For this review, take the finished solid that the model builds, in its own axes (mm). A direction names the side the tool comes from. Coordinates: 2 decimals unless noted, no trailing zeros. Write each loop counter-clockwise with the first axis right and the second up, starting at its lowest first coordinate (ties: lowest second). Pieces come first, ordered by that corner, then holes.
1) To check wall thickness, follow line 1 along Z through (x, y) = (7, 14); line 2 along Z through (x, y) = (-6, -3.5); line 3 along X through (y, z) = (-0.5, 7). State the ranges of each line that lie inside material, in increasing order.
2) Mouldability with a two-part tool opening along Z and no side actions: class faces 3 (the face through (0, 25, -71)), 4 (the face through (0, 0, 24.9)), 5 (the face through (0, 0, -143)) as pulls with the +Z half, pulls with the -Z half, needs draft (parallel to the pull), parting line crosses it, or undercut.
3) We need section B-B on y = 7. Write out the cut boundary in (x, z).
4) For faces 1 (the face through (-11, 6, 0)), 2 (the face through (-25, 0, -71)), list the 3-axis set-ups (+Z, -Z, +X, -X, +Y, -Y) from which the entire face can be reached by the end or side of a thin tool; tool diameter is ignored.
5) We need section C-C on x = 15. Write out the cut boundary in (y, z), then the cut area to 3 significant figures.
6) Insertion check: P1, Ø1, axis at y = 7, z = 2, coming from the +X side; P2, Ø1.5, axis at x = 8, y = -16.5, coming from the +Z side; P3, Ø8, axis at x = -10, z = 3.5, coming from the -Y side. Each pin has a flat end and moves straight along its axis. Give the tip position at first contact, or say it passes through.
7) We need section A-A on x = 0. Write out the cut boundary in (y, z).
Autodesk Inventor part; units mm, degrees
ref_plane "YZ Plane" through (0, 0, 0) normal (1, 0, 0) x (0, 1, 0)
ref_plane "XZ Plane" through (0, 0, 0) normal (0, 1, 0) x (-1, 0, 0)
ref_plane "XY Plane" through (0, 0, 0) normal (0, 0, 1) x (1, 0, 0)
sketch "Sketch1" plane through (0, 0, 0) normal (0, 0, 1) x (1, 0, 0)
  line L0 (-25, 25) -> (25, 25)
  line L1 (25, 25) -> (25, -25)
  line L2 (25, -25) -> (-25, -25)
  line L3 (-25, -25) -> (-25, 25)
  point P0 (0, 0)
  dimension "d0" = 50
  dimension "d1" = 50
  dimension "d2" = 25
  dimension "d3" = 25
extrude "Extrusion1" add sketch "Sketch1" against normal blind 143
sketch "Sketch2" plane through (0, 0, 0) normal (0, 0, 1) x (1, 0, 0)
  circle A0 centre (0, 0) radius 11
  dimension "d7" = 22
extrude "Extrusion2" add sketch "Sketch2" along normal blind 2.4
sketch "Sketch3" plane through (0, 0, 2.4) normal (0, 0, 1) x (1, 0, 0)
  circle A0 centre (0, 0) radius 4
  dimension "d10" = 8
extrude "Extrusion3" add sketch "Sketch3" along normal blind 22.5
fillet "Fillet1" radius 2 4 edges at (-25, 25, -71.5) (25, 25, -71.5) (25, -25, -71.5) (-25, -25, -71.5)
fillet "Fillet2" radius 1 8 edges at (-24.4142, 24.4142, 0) (-25, 0, 0) (-24.4142, -24.4142, 0) (0, -25, 0) (24.4142, -24.4142, 0) (25, 0, 0) (24.4142, 24.4142, 0) (0, 25, 0)
properties part number "Electric Motor"
Result:
1. line 1: z = -143 to 0
1. line 2: z = -143 to 2.4
1. line 3: x = -3.97 to 3.97
2. face 3: needs draft
2. face 4: pulls with the +Z half
2. face 5: pulls with the -Z half
3. outline: (-25, -143) - (25, -143) - (25, -1) arc R1 ccw to (24, 0) - (8.49, 0) - (8.49, 2.4) - (-8.49, 2.4) - (-8.49, 0) - (-24, 0) arc R1 ccw to (-25, -1) - close
4. face 1: +Z
4. face 2: +Z, -Z, -X, +Y, -Y
5. outline: (-25, -143) - (25, -143) - (25, -1) arc R1 ccw to (24, 0) - (-24, 0) arc R1 ccw to (-25, -1) - close
5. area: 7,150 mm2
6. P1: stops at x = 8.87
6. P2: stops at z = 0
6. P3: stops at y = -24.87
7. outline: (-25, -143) - (25, -143) - (25, -1) arc R1 ccw to (24, 0) - (11, 0) - (11, 2.4) - (4, 2.4) - (4, 24.9) - (-4, 24.9) - (-4, 2.4) - (-11, 2.4) - (-11, 0) - (-24, 0) arc R1 ccw to (-25, -1) - close
